The figure shows three views and two pictorial views of one solid part (mm, origin at its lowest corner). Answer the questions. A direction names the side the tool comes from. Coordinates: 2 decimals unless noted, no trailing zeros. Order: outer loops, then holes, each group sorted by start corner. A loop starts at its lowest first (then second) coordinate and runs counter-clockwise, first axis right, second up. Notation, with made-up numbers: (42, 12.25) - (92, 12.25) arc R31 ccw to (92, 45.25) - close; hole circle Ø11 at (68.25, 25). An arc over 180 degrees is marked (long way). Use one line per item in the form item = value. Start each with the question number.
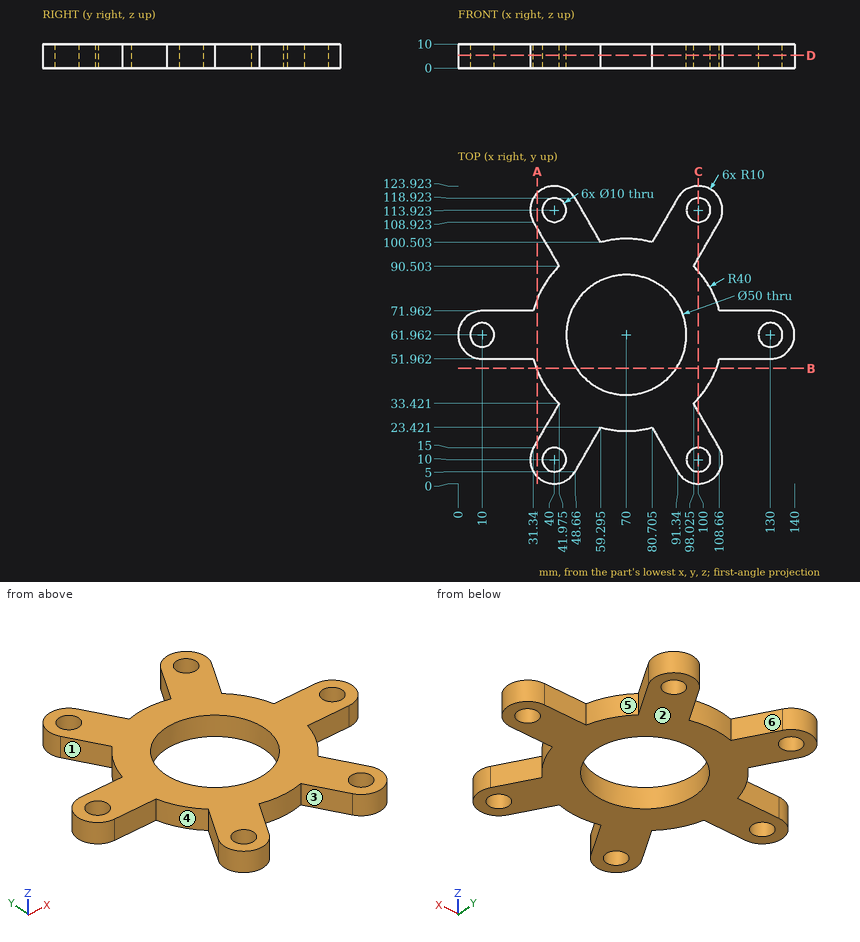
Q1. A cutting plane is placed at C-C (x = 100). Give the vertices of the cut face in (y, z) (1 decimal).
Q2. Given P1, Ø3, axis at x = 116, z = 7, coming from the -Y side; P2, Ø3, axis at y = 70, z = 1, coming from the -X side (1 decimal); P3, Ø3, axis at x = 104.5, z = 1, coming from the -Y side, each flat-ended and moving along its own axis, determine where each tip first touches the part or whether it passes through.
Q3. A cutting plane is placed at D-D (z = 5.25). Give the number of separate pieces and of enclosed holes in the cut face.
Q4. A cutting plane is placed at A-A (x = 33). Give the vertices of the cut face in (y, z) (1 decimal).
Q5. Consider probe 1 along Y at (x, z) = (100, 4) (1 decimal); probe 2 along Y at (x, z) = (10, 4); probe 3 along Y at (x, z) = (70, 4). Determine where each line is inside the solid, lowest interval first.
Q6. A cutting plane is placed at B-B (y = 48). Give the vertices of the cut face in (x, z) (1 decimal).
Q7. Which of the six approach directions +Z, -Z, +X, -X, +Y, -Y give full straight-line access (tool end or side, diameter ignored) to the marked faces 4, 5 and 6?
Q8. For a pull along X with two mould halves and no side action, classify the marked faces 1, 2 and 3 as +X half, -X half, draft (parallel to the pull), parting line (faces both ways), or undercut.
Result sheet:
q1.outline = (0, 0) - (5, 0) - (5, 10) - (0, 10) - close; (15, 0) - (30, 0) - (30, 10) - (15, 10) - close; (35.5, 0) - (88.4, 0) - (88.4, 10) - (35.5, 10) - close; (93.9, 0) - (108.9, 0) - (108.9, 10) - (93.9, 10) - close; (118.9, 0) - (123.9, 0) - (123.9, 10) - (118.9, 10) - close
q2.P1 = 51.96
q2.P2 = 2.4
q2.P3 = 0.46
q3.separate_pieces = 1
q3.enclosed_holes = 7
q4.outline = (2.9, 0) - (17.9, 0) - (17.9, 10) - (2.9, 10) - close; (46.8, 0) - (77.2, 0) - (77.2, 10) - (46.8, 10) - close; (106, 0) - (121.1, 0) - (121.1, 10) - (106, 10) - close
q5.probe_1 = 0 to 5, 15 to 30, 35.5 to 88.4, 93.9 to 108.9, 118.9 to 123.9
q5.probe_2 = 51.96 to 56.96, 66.96 to 71.96
q5.probe_3 = 21.96 to 36.96, 86.96 to 101.96
q6.outline = (32.5, 0) - (49.3, 0) - (49.3, 10) - (32.5, 10) - close; (90.7, 0) - (107.5, 0) - (107.5, 10) - (90.7, 10) - close
q7.face_4 = +Z, -Z, -X
q7.face_5 = +Z, -Z, +X
q7.face_6 = +Z, -Z, +Y
q8.face_1 = -X half
q8.face_2 = draft
q8.face_3 = undercut
